Part model, mm, in its own coordinate system. Give positions to 0.01 mm unless a question says otherwise; leave off trailing zeros. Answer in a Markdown table with one row per item.
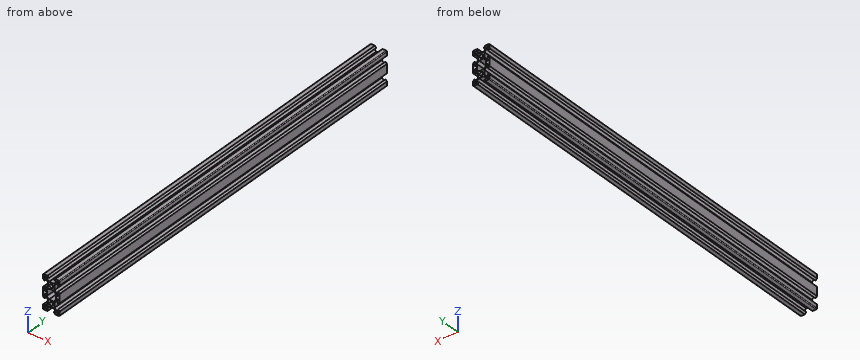
from build123d import *

# Parameters (mm, degrees)
F0_R     = 2.0955
F2_DEPTH = 500


with BuildPart() as f2:
    # F0 (on Front) → F2 (new body)
    with BuildSketch(Plane.XZ):
        with BuildLine():
            ThreePointArc((-9.9949, -9.0043), (-9.7047599774, -9.7047599774), (-9.0043, -9.9949))
            Line((-9.0043, -9.9949), (-4.6246692655, -9.9949))
            Line((-4.6246692655, -9.9949), (-2.8212692655, -8.1915))
            Line((-2.8212692655, -8.1915), (-5.4628692655, -8.1915))
            Line((-5.4628692655, -8.1915), (-5.4628692655, -6.5405))
            Line((-5.4628692655, -6.5405), (-2.8212692655, -3.8989))
            Line((-2.8212692655, -3.8989), (2.8212692655, -3.8989))
            Line((2.8212692655, -3.8989), (5.4628692655, -6.5405))
            Line((5.4628692655, -6.5405), (5.4628692655, -8.1915))
            Line((5.4628692655, -8.1915), (2.8212692655, -8.1915))
            Line((2.8212692655, -8.1915), (4.6246692655, -9.9949))
            Line((4.6246692655, -9.9949), (9.0043, -9.9949))
            ThreePointArc((9.0043, -9.9949), (9.7047599774, -9.7047599774), (9.9949, -9.0043))
            Line((9.9949, -9.0043), (9.9949, -4.6246692655))
            Line((9.9949, -4.6246692655), (8.1915, -2.8212692655))
            Line((8.1915, -2.8212692655), (8.1915, -5.4628692655))
            Line((8.1915, -5.4628692655), (6.5405, -5.4628692655))
            Line((6.5405, -5.4628692655), (3.8989, -2.8212692655))
            Line((3.8989, -2.8212692655), (3.8989, 2.8212692655))
            Line((3.8989, 2.8212692655), (6.5405, 5.4628692655))
            Line((6.5405, 5.4628692655), (8.1915, 5.4628692655))
            Line((8.1915, 5.4628692655), (8.1915, 2.8212692655))
            Line((8.1915, 2.8212692655), (9.9949, 4.6246692655))
            Line((9.9949, 4.6246692655), (9.9949, 9.0043))
            Line((9.9949, 9.0043), (9.9949, 10.9855))
            Line((9.9949, 10.9855), (9.9949, 15.3651307345))
            Line((9.9949, 15.3651307345), (8.1915, 17.1685307345))
            Line((8.1915, 17.1685307345), (8.1915, 14.5269307345))
            Line((8.1915, 14.5269307345), (6.5405, 14.5269307345))
            Line((6.5405, 14.5269307345), (3.8989, 17.1685307345))
            Line((3.8989, 17.1685307345), (3.8989, 22.8110692655))
            Line((3.8989, 22.8110692655), (6.5405, 25.4526692655))
            Line((6.5405, 25.4526692655), (8.1915, 25.4526692655))
            Line((8.1915, 25.4526692655), (8.1915, 22.8110692655))
            Line((8.1915, 22.8110692655), (9.9949, 24.6144692655))
            Line((9.9949, 24.6144692655), (9.9949, 28.9941))
            ThreePointArc((9.9949, 28.9941), (9.7047599774, 29.6945599774), (9.0043, 29.9847))
            Line((9.0043, 29.9847), (4.6246692655, 29.9847))
            Line((4.6246692655, 29.9847), (2.8212692655, 28.1813))
            Line((2.8212692655, 28.1813), (5.4628692655, 28.1813))
            Line((5.4628692655, 28.1813), (5.4628692655, 26.5303))
            Line((5.4628692655, 26.5303), (2.8212692655, 23.8887))
            Line((2.8212692655, 23.8887), (-2.8212692655, 23.8887))
            Line((-2.8212692655, 23.8887), (-5.4628692655, 26.5303))
            Line((-5.4628692655, 26.5303), (-5.4628692655, 28.1813))
            Line((-5.4628692655, 28.1813), (-2.8212692655, 28.1813))
            Line((-2.8212692655, 28.1813), (-4.6246692655, 29.9847))
            Line((-4.6246692655, 29.9847), (-9.0043, 29.9847))
            ThreePointArc((-9.0043, 29.9847), (-9.7047599774, 29.6945599774), (-9.9949, 28.9941))
            Line((-9.9949, 28.9941), (-9.9949, 24.6144692655))
            Line((-9.9949, 24.6144692655), (-8.1915, 22.8110692655))
            Line((-8.1915, 22.8110692655), (-8.1915, 25.4526692655))
            Line((-8.1915, 25.4526692655), (-6.5405, 25.4526692655))
            Line((-6.5405, 25.4526692655), (-3.8989, 22.8110692655))
            Line((-3.8989, 22.8110692655), (-3.8989, 17.1685307345))
            Line((-3.8989, 17.1685307345), (-6.5405, 14.5269307345))
            Line((-6.5405, 14.5269307345), (-8.1915, 14.5269307345))
            Line((-8.1915, 14.5269307345), (-8.1915, 17.1685307345))
            Line((-8.1915, 17.1685307345), (-9.9949, 15.3651307345))
            Line((-9.9949, 15.3651307345), (-9.9949, 10.9855))
            Line((-9.9949, 10.9855), (-9.9949, 9.0043))
            Line((-9.9949, 9.0043), (-9.9949, 4.6246692655))
            Line((-9.9949, 4.6246692655), (-8.1915, 2.8212692655))
            Line((-8.1915, 2.8212692655), (-8.1915, 5.4628692655))
            Line((-8.1915, 5.4628692655), (-6.5405, 5.4628692655))
            Line((-6.5405, 5.4628692655), (-3.8989, 2.8212692655))
            Line((-3.8989, 2.8212692655), (-3.8989, -2.8212692655))
            Line((-3.8989, -2.8212692655), (-6.5405, -5.4628692655))
            Line((-6.5405, -5.4628692655), (-8.1915, -5.4628692655))
            Line((-8.1915, -5.4628692655), (-8.1915, -2.8212692655))
            Line((-8.1915, -2.8212692655), (-9.9949, -4.6246692655))
            Line((-9.9949, -4.6246692655), (-9.9949, -9.0043))
        make_face()
        with BuildLine():
            ThreePointArc((-8.0391, -8.1915), (-8.1468630735, -8.1468630735), (-8.1915, -8.0391))
            Line((-8.1915, -8.0391), (-8.1915, -6.6929))
            ThreePointArc((-8.1915, -6.6929), (-8.1468630735, -6.5851369265), (-8.0391, -6.5405))
            Line((-8.0391, -6.5405), (-7.9883, -6.5405))
            Line((-7.9883, -6.5405), (-6.5405, -7.9883))
            Line((-6.5405, -7.9883), (-6.5405, -8.0391))
            ThreePointArc((-6.5405, -8.0391), (-6.5851369265, -8.1468630735), (-6.6929, -8.1915))
            Line((-6.6929, -8.1915), (-8.0391, -8.1915))
        make_face(mode=Mode.SUBTRACT)
        with BuildLine():
            Line((-7.9883, 6.5405), (-8.0391, 6.5405))
            ThreePointArc((-8.0391, 6.5405), (-8.1468630735, 6.5851369265), (-8.1915, 6.6929))
            Line((-8.1915, 6.6929), (-8.1915, 8.0391))
            ThreePointArc((-8.1915, 8.0391), (-8.1468630735, 8.1468630735), (-8.0391, 8.1915))
            Line((-8.0391, 8.1915), (-6.6929, 8.1915))
            ThreePointArc((-6.6929, 8.1915), (-6.5851369265, 8.1468630735), (-6.5405, 8.0391))
            Line((-6.5405, 8.0391), (-6.5405, 7.9883))
            Line((-6.5405, 7.9883), (-7.9883, 6.5405))
        make_face(mode=Mode.SUBTRACT)
        with BuildLine():
            Line((8.1915, -6.6929), (8.1915, -8.0391))
            ThreePointArc((8.1915, -8.0391), (8.1468630735, -8.1468630735), (8.0391, -8.1915))
            Line((8.0391, -8.1915), (6.6929, -8.1915))
            ThreePointArc((6.6929, -8.1915), (6.5851369265, -8.1468630735), (6.5405, -8.0391))
            Line((6.5405, -8.0391), (6.5405, -7.9883))
            Line((6.5405, -7.9883), (7.9883, -6.5405))
            Line((7.9883, -6.5405), (8.0391, -6.5405))
            ThreePointArc((8.0391, -6.5405), (8.1468630735, -6.5851369265), (8.1915, -6.6929))
        make_face(mode=Mode.SUBTRACT)
        Circle(F0_R, mode=Mode.SUBTRACT)
        with BuildLine():
            ThreePointArc((8.1915, 6.6929), (8.1468630735, 6.5851369265), (8.0391, 6.5405))
            Line((8.0391, 6.5405), (7.9883, 6.5405))
            Line((7.9883, 6.5405), (6.5405, 7.9883))
            Line((6.5405, 7.9883), (6.5405, 8.0391))
            ThreePointArc((6.5405, 8.0391), (6.5851369265, 8.1468630735), (6.6929, 8.1915))
            Line((6.6929, 8.1915), (8.0391, 8.1915))
            ThreePointArc((8.0391, 8.1915), (8.1468630735, 8.1468630735), (8.1915, 8.0391))
            Line((8.1915, 8.0391), (8.1915, 6.6929))
        make_face(mode=Mode.SUBTRACT)
        with BuildLine():
            ThreePointArc((-8.1915, 13.2969), (-8.1468630735, 13.4046630735), (-8.0391, 13.4493))
            Line((-8.0391, 13.4493), (-7.9883, 13.4493))
            Line((-7.9883, 13.4493), (-6.5405, 12.0015))
            Line((-6.5405, 12.0015), (-6.5405, 11.9507))
            ThreePointArc((-6.5405, 11.9507), (-6.5851369265, 11.8429369265), (-6.6929, 11.7983))
            Line((-6.6929, 11.7983), (-8.0391, 11.7983))
            ThreePointArc((-8.0391, 11.7983), (-8.1468630735, 11.8429369265), (-8.1915, 11.9507))
            Line((-8.1915, 11.9507), (-8.1915, 13.2969))
        make_face(mode=Mode.SUBTRACT)
        with BuildLine():
            ThreePointArc((-6.6929, 28.1813), (-6.5851369265, 28.1366630735), (-6.5405, 28.0289))
            Line((-6.5405, 28.0289), (-6.5405, 27.9781))
            Line((-6.5405, 27.9781), (-7.9883, 26.5303))
            Line((-7.9883, 26.5303), (-8.0391, 26.5303))
            ThreePointArc((-8.0391, 26.5303), (-8.1468630735, 26.5749369265), (-8.1915, 26.6827))
            Line((-8.1915, 26.6827), (-8.1915, 28.0289))
            ThreePointArc((-8.1915, 28.0289), (-8.1468630735, 28.1366630735), (-8.0391, 28.1813))
            Line((-8.0391, 28.1813), (-6.6929, 28.1813))
        make_face(mode=Mode.SUBTRACT)
        Polygon((5.4628692655, 6.5405), (2.8212692655, 3.8989), (-2.8212692655, 3.8989), (-5.4628692655, 6.5405), (-5.4628692655, 13.4493), (-2.8212692655, 16.0909), (2.8212692655, 16.0909), (5.4628692655, 13.4493), align=None, mode=Mode.SUBTRACT)
        with Locations((0, 19.9898)):
            Circle(F0_R, mode=Mode.SUBTRACT)
        with BuildLine():
            Line((8.0391, 11.7983), (6.6929, 11.7983))
            ThreePointArc((6.6929, 11.7983), (6.5851369265, 11.8429369265), (6.5405, 11.9507))
            Line((6.5405, 11.9507), (6.5405, 12.0015))
            Line((6.5405, 12.0015), (7.9883, 13.4493))
            Line((7.9883, 13.4493), (8.0391, 13.4493))
            ThreePointArc((8.0391, 13.4493), (8.1468630735, 13.4046630735), (8.1915, 13.2969))
            Line((8.1915, 13.2969), (8.1915, 11.9507))
            ThreePointArc((8.1915, 11.9507), (8.1468630735, 11.8429369265), (8.0391, 11.7983))
        make_face(mode=Mode.SUBTRACT)
        with BuildLine():
            ThreePointArc((6.5405, 28.0289), (6.5851369265, 28.1366630735), (6.6929, 28.1813))
            Line((6.6929, 28.1813), (8.0391, 28.1813))
            ThreePointArc((8.0391, 28.1813), (8.1468630735, 28.1366630735), (8.1915, 28.0289))
            Line((8.1915, 28.0289), (8.1915, 26.6827))
            ThreePointArc((8.1915, 26.6827), (8.1468630735, 26.5749369265), (8.0391, 26.5303))
            Line((8.0391, 26.5303), (7.9883, 26.5303))
            Line((7.9883, 26.5303), (6.5405, 27.9781))
            Line((6.5405, 27.9781), (6.5405, 28.0289))
        make_face(mode=Mode.SUBTRACT)
    extrude(amount=F2_DEPTH)


solid = f2.part
(1) Saw through at A-A (y = -219.5). Give the number of separate pieces and of enclosed holes in the cut face, plus the area to 3 significant figures.
Recorded:
| item | result |
|---|---|
| separate pieces | 1 |
| enclosed holes | 11 |
| area | 318 mm^2 |
(2) Pin check, flat tips, straight feed: pin 1 Ø3 at (x, y) = (-1, -361) entering from -Z; pin 2 Ø3 at (y, z) = (-321.5, 18.5) entering from -X; pin 3 Ø3 at (x, y) = (2.5, -165) entering from +Z. Stop position of each tip, or through.
Recorded:
| item | result |
|---|---|
| pin 1 | stops at z = -3.9 |
| pin 2 | stops at x = -8.36 |
| pin 3 | stops at z = 29.36 |
(3) Drill centre lines: line 1 along Z through (x, y) = (0, -368); line 2 along Z through (x, y) = (5.75, -344.5); line 3 along Z through (x, y) = (-8.25, -138.5). Where is each one in solid material? Low to high.
Recorded:
| item | result |
|---|---|
| line 1 | z = -3.9 to -2.1, 2.1 to 3.9, 16.09 to 17.89, 22.09 to 23.89 |
| line 2 | z = -9.99 to -4.67, 4.67 to 15.32, 24.66 to 29.98 |
| line 3 | z = -9.99 to -2.88, 2.88 to 17.11, 22.87 to 29.98 |
